Read the model definition and answer for the solid it produces. Units are mm, in the model's axes. Face numbers are marked on the shaded views. A direction names the side the tool comes from. Give positions to 0.01 mm unless a question says otherwise; leave off trailing zeros. Loops run counter-clockwise (first coordinate to the right, second up) from the corner with the lowest first, then second, coordinate; pieces in that order, holes last. Notation, with made-up numbers: (-36.5, -34.75) - (-23.5, -34.75) arc R15 cw to (-23.5, -19.75) - close; hole circle Ø6 at (-11, 15.25). An arc over 180 degrees is marked (long way). Put each result on its own line as item: value. Start each with the question number.
1. A cutting plane is placed at C-C, the plane z = 12.25. Count the separate pieces of the cut face and the enclosed holes in it, plus the area to 3 significant figures.
2. A cutting plane is placed at D-D, the plane x = 23.5. Determine the outline of the cut face in (y, z), plus the area to 3 significant figures.
3. Given pin 1 Ø1.5 at (x, y) = (34, 19) entering from +Z; pin 2 Ø1.5 at (y, z) = (31.5, 6.5) entering from +X; pin 3 Ø0.9 at (y, z) = (6, 12.5) entering from +X, each flat-ended and moving along its own axis, determine where each tip first touches the part or whether it passes through.
4. A cutting plane is placed at B-B, the plane x = 5.5. Determine the outline of the cut face in (y, z), plus the area to 3 significant figures.
5. For the marked faces 5, 6 and 7, determine the directions among +Z, -Z, +X, -X, +Y, -Y from which every point of the face is accessible in a straight line to the end or side of a thin tool.
6. Consider L1, parallel to X at y = 19, z = 9.5; L2, parallel to X at y = 26, z = 3.5. Determine where each line is inside the solid, lowest interval first. Write a range as from..to.
7. A cutting plane is placed at A-A, the plane y = 5.5. Determine the outline of the cut face in (x, z), plus the area to 3 significant figures.
8. For a pull along X with two mould halves and no side action, classify the marked faces 1, 2, 3 and 4 as released by +X, released by -X, zero draft, split by the parting line, or undercut.
```python
from build123d import *

# Parameters (mm, degrees)
SKETCH1_W           = 42
SKETCH1_H           = 42
BOSS_EXTRUDE1_DEPTH = 16
CUT_EXTRUDE2_DEPTH  = 13
FILLET2_R           = 1
FILLET3_R           = 4
FILLET4_R           = 4
FILLET6_R           = 4
FILLET8_R           = 2
FILLET9_R           = 2
FILLET11_R          = 2
FILLET12_R          = 2
FILLET13_R          = 2
CUT_EXTRUDE3_REACH  = 63.514
SKETCH4_R           = 1.6
SKETCH4_R_2         = 3.6
SKETCH5_W           = 11.093459678
SKETCH5_H           = 7
SKETCH5_W_2         = 7
CUT_EXTRUDE14_DEPTH = 13
FILLET14_R          = 2
FILLET15_R          = 2
FILLET16_R          = 2
FILLET17_R          = 2
FILLET18_R          = 2
FILLET19_R          = 2
FILLET20_R          = 2
FILLET21_R          = 2
FILLET22_R          = 2
FILLET23_R          = 2
FILLET24_R          = 2
FILLET25_R          = 2
FILLET26_R          = 2


with BuildPart() as part:
    # Sketch1 → Boss-Extrude1 (new body)
    with BuildSketch(Plane.XY):
        with Locations((21, 21)):
            Rectangle(SKETCH1_W, SKETCH1_H)
    extrude(amount=BOSS_EXTRUDE1_DEPTH)

    # Sketch3 → Cut-Extrude2 (cut)
    with BuildSketch(Plane.XY.offset(16)):
        Polygon((39, 42), (39, 39), (42, 39), (42, 36), (36, 36), (36, 42), align=None)
        Polygon((33, 42), (33, 33), (42, 33), (42, 30), (30, 30), (30, 42), align=None)
        Polygon((42, 27), (27, 27), (27, 42), (24, 42), (24, 24), (42, 24), align=None)
        Polygon((42, 21), (21, 21), (21, 42), (18, 42), (18, 18), (42, 18), align=None)
        Polygon((42, 14), (14, 14), (14, 42), (11, 42), (11, 11), (42, 11), align=None)
        Polygon((42, 7), (7, 7), (7, 42), (4, 42), (4, 4), (42, 4), align=None)
    extrude(amount=-CUT_EXTRUDE2_DEPTH, mode=Mode.SUBTRACT)

    # Fillet2
    fillet2_edges = [part.edges().sort_by_distance(p)[0] for p in [
        (39, 39, 9.5),
    ]]
    fillet(fillet2_edges, radius=FILLET2_R)

    # Fillet3
    fillet3_edges = [part.edges().sort_by_distance(p)[0] for p in [
        (33, 33, 9.5),
    ]]
    fillet(fillet3_edges, radius=FILLET3_R)

    # Fillet4
    fillet4_edges = [part.edges().sort_by_distance(p)[0] for p in [
        (27, 27, 9.5),
    ]]
    fillet(fillet4_edges, radius=FILLET4_R)

    # Fillet6
    fillet6_edges = [part.edges().sort_by_distance(p)[0] for p in [
        (14, 14, 9.5),
    ]]
    fillet(fillet6_edges, radius=FILLET6_R)

    # Fillet8
    fillet8_edges = [part.edges().sort_by_distance(p)[0] for p in [
        (36, 36, 9.5),
    ]]
    fillet(fillet8_edges, radius=FILLET8_R)

    # Fillet9
    fillet9_edges = [part.edges().sort_by_distance(p)[0] for p in [
        (30, 30, 9.5),
    ]]
    fillet(fillet9_edges, radius=FILLET9_R)

    # Fillet11
    fillet11_edges = [part.edges().sort_by_distance(p)[0] for p in [
        (18, 18, 9.5),
    ]]
    fillet(fillet11_edges, radius=FILLET11_R)

    # Fillet12
    fillet12_edges = [part.edges().sort_by_distance(p)[0] for p in [
        (11, 11, 9.5),
    ]]
    fillet(fillet12_edges, radius=FILLET12_R)

    # Fillet13
    fillet13_edges = [part.edges().sort_by_distance(p)[0] for p in [
        (4, 4, 9.5),
    ]]
    fillet(fillet13_edges, radius=FILLET13_R)

    # Sketch4 → Cut-Extrude3 (cut, up to next)
    with BuildSketch(Plane(origin=(0, 0, 0), x_dir=(-1, 0, 0), z_dir=(0, 0, -1)), mode=Mode.PRIVATE) as cut_extrude3_sk1:
        with Locations((-36.5, 5.5)):
            Circle(SKETCH4_R)
    cut_extrude3_tool1 = extrude(cut_extrude3_sk1.sketch, amount=-CUT_EXTRUDE3_REACH, mode=Mode.PRIVATE) & part.part
    # Sketch4 → Cut-Extrude3 (cut, up to next)
    with BuildSketch(Plane(origin=(0, 0, 0), x_dir=(-1, 0, 0), z_dir=(0, 0, -1)), mode=Mode.PRIVATE) as cut_extrude3_sk2:
        with Locations((-5.5, 5.5)):
            Circle(SKETCH4_R)
    cut_extrude3_tool2 = extrude(cut_extrude3_sk2.sketch, amount=-CUT_EXTRUDE3_REACH, mode=Mode.PRIVATE) & part.part
    # Sketch4 → Cut-Extrude3 (cut, up to next)
    with BuildSketch(Plane(origin=(0, 0, 0), x_dir=(-1, 0, 0), z_dir=(0, 0, -1)), mode=Mode.PRIVATE) as cut_extrude3_sk3:
        with Locations((-21, 21)):
            Circle(SKETCH4_R_2)
    cut_extrude3_tool3 = extrude(cut_extrude3_sk3.sketch, amount=-CUT_EXTRUDE3_REACH, mode=Mode.PRIVATE) & part.part
    add(cut_extrude3_tool1.solids().sort_by_distance((36.5, 5.5, 0))[0], mode=Mode.SUBTRACT)
    add(cut_extrude3_tool2.solids().sort_by_distance((5.5, 5.5, 0))[0], mode=Mode.SUBTRACT)
    add(cut_extrude3_tool3.solids().sort_by_distance((21, 21, 0))[0], mode=Mode.SUBTRACT)

    # Sketch5 → Cut-Extrude14 (cut)
    with BuildSketch(Plane.XY.offset(16)):
        with Locations((36.5, 5.5)):
            Rectangle(SKETCH5_W, SKETCH5_H)
        with Locations((5.5, 5.5)):
            Rectangle(SKETCH5_W_2, SKETCH5_H)
    extrude(amount=-CUT_EXTRUDE14_DEPTH, mode=Mode.SUBTRACT)

    # Fillet14
    fillet14_edges = [part.edges().sort_by_distance(p)[0] for p in [
        (24, 24, 9.5),
    ]]
    fillet(fillet14_edges, radius=FILLET14_R)

    # Fillet15
    fillet15_edges = [part.edges().sort_by_distance(p)[0] for p in [
        (9, 2, 9.5),
    ]]
    fillet(fillet15_edges, radius=FILLET15_R - 0.0001)  # a hair under: the kernel refuses the full size

    # Fillet16
    fillet16_edges = [part.edges().sort_by_distance(p)[0] for p in [
        (2, 2, 9.5),
    ]]
    fillet(fillet16_edges, radius=FILLET16_R)

    # Fillet17
    fillet17_edges = [part.edges().sort_by_distance(p)[0] for p in [
        (2, 9, 9.5),
    ]]
    fillet(fillet17_edges, radius=FILLET17_R - 0.0001)  # a hair under: the kernel refuses the full size

    # Fillet18
    fillet18_edges = [part.edges().sort_by_distance(p)[0] for p in [
        (9, 9, 9.5),
    ]]
    fillet(fillet18_edges, radius=FILLET18_R - 0.0001)  # a hair under: the kernel refuses the full size

    # Fillet19
    fillet19_edges = [part.edges().sort_by_distance(p)[0] for p in [
        (4, 9, 9.5),
    ]]
    fillet(fillet19_edges, radius=FILLET19_R)

    # Fillet20
    fillet20_edges = [part.edges().sort_by_distance(p)[0] for p in [
        (7, 9, 9.5),
    ]]
    fillet(fillet20_edges, radius=FILLET20_R)

    # Fillet21
    fillet21_edges = [part.edges().sort_by_distance(p)[0] for p in [
        (9, 7, 9.5),
    ]]
    fillet(fillet21_edges, radius=FILLET21_R)

    # Fillet22
    fillet22_edges = [part.edges().sort_by_distance(p)[0] for p in [
        (9, 4, 9.5),
    ]]
    fillet(fillet22_edges, radius=FILLET22_R)

    # Fillet23
    fillet23_edges = [part.edges().sort_by_distance(p)[0] for p in [
        (30.953270161, 9, 9.5),
    ]]
    fillet(fillet23_edges, radius=FILLET23_R - 0.0001)  # a hair under: the kernel refuses the full size

    # Fillet24
    fillet24_edges = [part.edges().sort_by_distance(p)[0] for p in [
        (30.953270161, 7, 9.5),
    ]]
    fillet(fillet24_edges, radius=FILLET24_R)

    # Fillet25
    fillet25_edges = [part.edges().sort_by_distance(p)[0] for p in [
        (30.953270161, 4, 9.5),
    ]]
    fillet(fillet25_edges, radius=FILLET25_R - 0.0001)  # a hair under: the kernel refuses the full size

    # Fillet26
    fillet26_edges = [part.edges().sort_by_distance(p)[0] for p in [
        (30.953270161, 2, 9.5),
    ]]
    fillet(fillet26_edges, radius=FILLET26_R)


solid = part.part
```
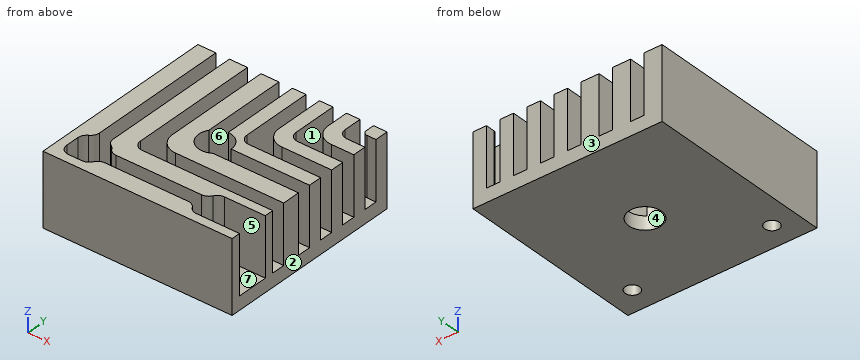
Return value:
1. separate pieces: 7
1. enclosed holes: 0
1. area: 954 mm2
2. outline: (0, 0) - (18.41, 0) - (18.41, 3) - (18, 3) - (18, 16) - (14, 16) - (14, 3) - (11, 3) - (11, 16) - (7, 16) - (7, 3) - (4, 3) - (4, 16) - (0, 16) - close; (23.59, 0) - (42, 0) - (42, 16) - (23.59, 16) - close
2. area: 506 mm2
3. pin 1: stops at z = 3
3. pin 2: stops at x = 30.44
3. pin 3: stops at x = 2
4. outline: (0, 0) - (3.9, 0) - (3.9, 3) - (2, 3) - (2, 16) - (0, 16) - close; (7.1, 0) - (42, 0) - (42, 3) - (7.1, 3) - close
4. area: 142 mm2
5. face 5: +Z, +X
5. face 6: +Z, +Y
5. face 7: +Z
6. L1: x = 0..4, 7..11, 14..18.01
6. L2: x = 0..4, 7..11, 14..18, 21..24
7. outline: (0, 0) - (3.9, 0) - (3.9, 3) - (2, 3) - (2, 16) - (0, 16) - close; (7.1, 0) - (34.9, 0) - (34.9, 3) - (7.1, 3) - close; (38.1, 0) - (42, 0) - (42, 3) - (38.1, 3) - close
7. area: 133 mm2
8. face 1: undercut
8. face 2: released by +X
8. face 3: zero draft
8. face 4: undercut
